Geometry check sheet. Reference: the model listing, model coordinates, mm. Face numbers are marked on the shaded views. A direction names the side the tool comes from. Coordinates: 2 decimals unless noted, no trailing zeros. Write each loop counter-clockwise with the first axis right and the second up, starting at its lowest first coordinate (ties: lowest second). Pieces come first, ordered by that corner, then holes.
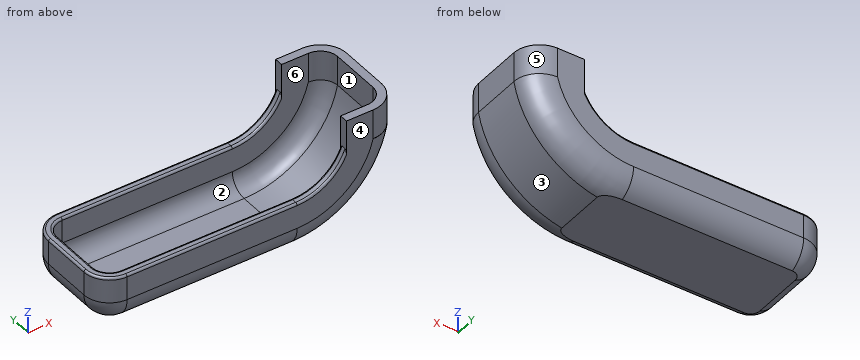
from build123d import *

# Parameters (mm, degrees)
F3_R      = 6
F4_T      = -2
F6_W      = 43.5708351433
F6_H      = 71.2567269802
F7_DEPTH  = 25.2
F9_DEPTH  = 7
F10_W     = 21.0461514253
F10_H     = 5.3538460713
F11_DEPTH = 73.3
F12_R     = 0.5


with BuildPart() as f2:
    # F2: sweep along a path in F0
    with BuildLine(Plane.XZ) as f2_path:
        Line((0, -24.4), (46, -24.4))
        ThreePointArc((46, -24.4), (61.6204993518, -18.7445992222), (70, -4.4))
    # F1 (on Right) → F2 (sweep)
    with BuildSketch(Plane.YZ):
        with BuildLine():
            Line((-6, -24.4), (6, -24.4))
            ThreePointArc((6, -24.4), (10.2426406871, -22.6426406871), (12, -18.4))
            Line((12, -18.4), (12, -12.4))
            Line((12, -12.4), (-12, -12.4))
            Line((-12, -12.4), (-12, -18.4))
            ThreePointArc((-12, -18.4), (-10.2426406871, -22.6426406871), (-6, -24.4))
        make_face()
    sweep(path=f2_path.line)

    # F3
    f3_edges = [f2.edges().sort_by_distance(p)[0] for p in [
        (0, -12, -15.4),
        (0, 10.242641, -22.642641),
        (0, 12, -15.4),
        (0, -10.242641, -22.642641),
    ]]
    fillet(f3_edges, radius=F3_R)

    # F4
    f4_openings = [f2.faces().sort_by_distance(p)[0] for p in [
        (23.307448, 0, -12.4),
        (53.938287, 0, -9.525944),
        (63.838518, 0, -3.270395),
    ]]
    offset(amount=F4_T, openings=f4_openings)

    # F6 (on face) → F7 (cut)
    with BuildSketch(Plane.XY.offset(-4.4)):
        with Locations((56.7423906177, -0.4439689219)):
            Rectangle(F6_W, F6_H)
    extrude(amount=F7_DEPTH, mode=Mode.SUBTRACT)

    # F8 (on face) → F9 (join)
    with BuildSketch(Plane.XY.offset(-4.4)):
        with BuildLine():
            Line((63.8661691473, 12), (57.593101397, 12))
            Line((57.593101397, 12), (57.593101397, 10))
            Line((57.593101397, 10), (63.8661691473, 10))
            ThreePointArc((63.8661691473, 10), (66.7292527517, 8.8342023924), (67.9636062613, 6))
            Line((67.9636062613, 6), (67.9636062613, -6))
            ThreePointArc((67.9636062613, -6), (66.7292527517, -8.8342023924), (63.8661691473, -10))
            Line((63.8661691473, -10), (57.593101397, -10))
            Line((57.593101397, -10), (57.593101397, -12))
            Line((57.593101397, -12), (63.8661691473, -12))
            ThreePointArc((63.8661691473, -12), (68.1563871176, -10.250588481), (70, -6))
            Line((70, -6), (70, 6))
            ThreePointArc((70, 6), (68.1563871176, 10.250588481), (63.8661691473, 12))
        make_face()
    extrude(amount=F9_DEPTH)

    # F10 (on face) → F11 (cut)
    with BuildSketch(Plane(origin=(0, 0, 0), x_dir=(0, -1, 0), z_dir=(-1, 0, 0))):
        with Locations((0.9807674214, -26.6769230357)):
            Rectangle(F10_W, F10_H)
    extrude(amount=-F11_DEPTH, mode=Mode.SUBTRACT)

    # F12
    f12_edges = [f2.edges().sort_by_distance(p)[0] for p in [
        (26, -12, -12.4),
        (53.042727, -12, -10.205881),
        (26, 12, -12.4),
        (1.757359, 10.242641, -12.4),
        (0, 0, -12.4),
        (1.757359, -10.242641, -12.4),
        (26, -10, -12.4),
        (3.171573, -8.828427, -12.4),
        (2, 0, -12.4),
        (3.171573, 8.828427, -12.4),
        (26, 10, -12.4),
        (53.042727, -10, -10.205881),
        (53.042727, 10, -10.205881),
        (53.042727, 12, -10.205881),
    ]]
    fillet(f12_edges, radius=F12_R)


solid = f2.part
1. Access from +Z, -Z, +X, -X, +Y, -Y to the whole of each face (thin tool, end or side, straight path). Record for the marked faces 1, 2 and 3.
Computed values:
face 1: +Z, -X
face 2: +Z
face 3: -Z, +X, +Y, -Y
2. Sectioned sample at A-A, the plane x = 16. Record the boundary of the cut face in (y, z), and give its area (3 significant figures).
Computed values:
outline: (-12, -18.4) arc R6 ccw to (-8.15, -24) - (8.15, -24) arc R6 ccw to (12, -18.4) - (12, -12.9) arc R0.5 ccw to (11.5, -12.4) - (10.5, -12.4) arc R0.5 ccw to (10, -12.9) - (10, -18.4) arc R4 cw to (6, -22.4) - (-6, -22.4) arc R4 cw to (-10, -18.4) - (-10, -12.9) arc R0.5 ccw to (-10.5, -12.4) - (-11.5, -12.4) arc R0.5 ccw to (-12, -12.9) - close
area: 73.2 mm2
3. Draft check along Y on the marked faces 4, 5 and 6. Enter one of: released by +Y, released by -Y, zero draft, split by the parting line, or undercut.
Computed values:
face 4: released by -Y
face 5: released by +Y
face 6: undercut
4. Gauge pin test, flat ends, axial feed: pin 1 Ø3.5 at (y, z) = (-1.5, -2.5) entering from -X; pin 2 Ø3 at (y, z) = (9.5, -13.5) entering from -X; pin 3 Ø5 at (y, z) = (8.5, -8.5) entering from +X. Record the tip position at first contact, or that the pin passes through.
Computed values:
pin 1: stops at x = 67.96
pin 2: stops at x = 0.34
pin 3: stops at x = 69.43
5. Sectioned sample at B-B, the plane z = -0.75. Record the boundary of the cut face in (x, y), and give its area (3 significant figures).
Computed values:
outline: (57.59, -12) - (63.87, -12) arc R6.14 ccw to (70, -6) - (70, 6) arc R6.14 ccw to (63.87, 12) - (57.59, 12) - (57.59, 10) - (63.87, 10) arc R4.1 cw to (67.96, 6) - (67.96, -6) arc R4.1 cw to (63.87, -10) - (57.59, -10) - close
area: 81.4 mm2
6. Thickness scan on line 1 along Y through (x, z) = (46, -18.75); line 2 along X through (y, z) = (3.75, -1); line 3 along Z through (x, y) = (39, -2.5). Record the ranges inside material, lowest first.
Computed values:
line 1: y = -11.99 to -9.98, 9.98 to 11.99
line 2: x = 67.96 to 70
line 3: z = -24 to -22.4
7. Sectioned sample at C-C, the plane y = 2. Record the boundary of the cut face in (x, z).
Computed values:
outline: (0, -18.4) arc R6 ccw to (3.85, -24) - (50.4, -24) arc R24.4 ccw to (70, -4.4) - (70, 2.6) - (67.96, 2.6) - (67.96, -4.4) arc R22.4 cw to (46, -22.4) - (6, -22.4) arc R4 cw to (2, -18.4) - (2, -12.9) arc R0.5 ccw to (1.5, -12.4) - (0.5, -12.4) arc R0.5 ccw to (0, -12.9) - close
